Autodesk Inventor part; units mm, degrees
ref_plane "YZ Plane" through (0, 0, 0) normal (1, 0, 0) x (0, 1, 0)
ref_plane "XZ Plane" through (0, 0, 0) normal (0, 1, 0) x (-1, 0, 0)
ref_plane "XY Plane" through (0, 0, 0) normal (0, 0, 1) x (1, 0, 0)
sketch "Sketch1" plane through (0, 0, 0) normal (0, 0, 1) x (1, 0, 0)
  line L0 (0, 0) -> (127, 0)
  line L1 (127, 0) -> (127, 76.2)
  line L2 (127, 76.2) -> (0, 76.2)
  line L3 (0, 76.2) -> (0, 0)
  line L4 (127, 76.2) -> (0, 76.2)
  line L5 (0, 76.2) -> (0, -889)
  line L6 (0, -889) -> (127, -889)
  line L7 (127, -889) -> (127, 76.2)
  dimension "d0" = 127
  dimension "d1" = 76.2
  dimension "d2" = 127
  dimension "d3" = 965.2
extrude "Extrusion1" add sketch "Sketch1" along normal blind 76.2
fillet "Fillet1" radius 31.75 2 edges at (127, -406.4, 0) (0, -406.4, 0)
sketch "Sketch2" plane through (0, 76.2, 76.2) normal (0, 1, 0) x (1, 0, 0)
  arc A0 (31.75, 76.2) -> (0, 44.45) centre (31.75, 44.45) ccw
  line L0 (0, 44.45) -> (0, 0)
  line L1 (127, 0) -> (0, 0)
  line L2 (127, 44.45) -> (127, 0)
  arc A1 (127, 44.45) -> (95.25, 76.2) centre (95.25, 44.45) ccw
  line L3 (95.25, 76.2) -> (31.75, 76.2)
  point P0 (0, 76.2)
extrude "Extrusion2" cut sketch "Sketch2" against normal blind 101.6
properties part number "BumperSide"
CAD build for the part. Positions are in the model's coordinates, mm. Round coordinates to 2 decimals unless told otherwise and drop trailing zeros. Loops run counter-clockwise (first coordinate to the right, second up) from the corner with the lowest first, then second, coordinate; pieces in that order, holes last.
(1) Wall check: line 1 along Z through (x, y) = (110, -422.5); line 2 along Z through (x, y) = (18.5, -538.5); line 3 along X through (y, z) = (-640.5, 19.5). Give the ranges that are in metal, low to high.
(2) Cut at B-B (x = 21). Give the cut face in (y, z).
(3) Cut at C-C (z = 11). Give the cut face in (x, y), plus the area to 3 significant figures.
(4) Cut at A-A (y = -656.5). Give the cut face in (x, z), plus the area to 3 significant figures.
(5) Drop flat-ended pins along their axis: pin 1 (8 mm diameter, centred on y = -603.5, z = 65, fed in from -X); pin 2 (4 mm diameter, centred on x = 22, y = -569.5, fed in from -Z); pin 3 (2 mm diameter, centred on x = 19.5, y = -530.5, fed in from -Z); pin 4 (4 mm diameter, centred on y = -200.5, z = 13.5, fed in from -X). Give the stop position or say it passes through.
Findings below:
1. line 1: z = 3.63 to 76.2
1. line 2: z = 2.9 to 76.2
1. line 3: x = 2.46 to 124.54
2. outline: (-889, 1.88) - (-25.4, 1.88) - (-25.4, 76.2) - (-889, 76.2) - close
3. outline: (7.72, -889) - (119.28, -889) - (119.28, -25.4) - (7.72, -25.4) - close
3. area: 96,300 mm2
4. outline: (0, 31.75) arc R31.75 ccw to (31.75, 0) - (95.25, 0) arc R31.75 ccw to (127, 31.75) - (127, 76.2) - (0, 76.2) - close
4. area: 9,240 mm2
5. pin 1: stops at x = 0
5. pin 2: stops at z = 0.96
5. pin 3: stops at z = 2.06
5. pin 4: stops at x = 4.47
